Source: CAD feature listing. Evaluate the final solid. Frame: model axes, mm. Face numbers are marked on the shaded views. A direction names the side the tool comes from. Coordinates: 2 decimals unless noted, no trailing zeros. Write each loop counter-clockwise with the first axis right and the second up, starting at its lowest first coordinate (ties: lowest second). Pieces come first, ordered by that corner, then holes. Notation, with made-up numbers: M -9,-3 L 11,-3 A12 ccw 11,12 Z; hole C -35.75,35 d2. An arc over 180 degrees is marked long. One line per item, written item: value. Start each with the question number.
Item 1: Pin query (flat end, axial travel): P1, Ø16, axis at x = -87.5, z = -8.5, coming from the +Y side; P2, Ø4, axis at x = -16.5, y = -41, coming from the +Z side; P3, Ø10, axis at y = -73.5, z = -13, coming from the -X side. Return the tip coordinate at first contact, or that it passes through.
Item 2: Mould query, pull axis X, two halves, no side actions, for the marked faces 5, 6 and 7. Classes: released by +X, released by -X, zero draft, split by the parting line, or undercut.
Item 3: Cut plane C-C, the plane y = -43.5. Output: boundary loops of the cut face in (x, z).
Item 4: Set-up query: the marked faces 1, 2, 3 and 4. Return all of +Z, -Z, +X, -X, +Y, -Y with unobstructed straight access to the full face (end or side cutting, diameter ignored); none if empty.
Item 5: Cut plane A-A, the plane z = 20. Output: boundary loops of the cut face in (x, y).
Item 6: Ray query, L1, parallel to Z at x = -65, y = -5.5; L2, parallel to Z at x = -65, y = -4; L3, parallel to Z at x = -113.5, y = -14. Return the intervals inside material, ascending. Write a range as from..to.
Item 7: Cut plane D-D, the plane x = -113. Output: boundary loops of the cut face in (y, z), then the cut area to 3 significant figures.
Item 8: Cut plane B-B, the plane x = -88. Output: boundary loops of the cut face in (y, z), then the cut area to 3 significant figures.
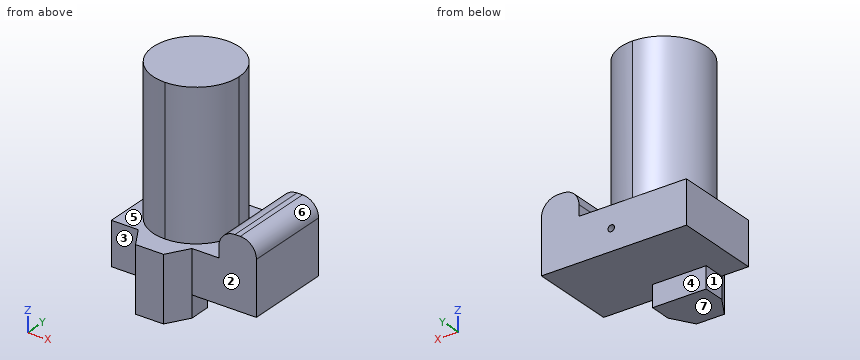
```python
from build123d import *

# Parameters (mm, degrees)
F1_DEPTH = 80
F3_DEPTH = 135
F5_DEPTH = 60
F6_R     = 3
F7_DEPTH = 10


# Not quite as in the source:
# - a feature names something its author has since deleted; it is built from what else it names


with BuildPart() as f1:
    # F0 (on Front) → F1 (new body)
    with BuildSketch(Plane.XZ):
        with BuildLine():
            Line((-135, 0), (0, 0))
            Line((0, 0), (0, 50))
            ThreePointArc((0, 50), (-4.3933982822, 60.6066017178), (-15, 65))
            Line((-15, 65), (-20, 65))
            ThreePointArc((-20, 65), (-30.6066017178, 60.6066017178), (-35, 50))
            Line((-35, 50), (-35, 40))
            Line((-35, 40), (-135, 40))
            Line((-135, 40), (-135, 0))
        make_face()
    extrude(amount=F1_DEPTH)

    # F2 (on face) → F3 (join)
    with BuildSketch(Plane.XY.offset(40)):
        with BuildLine():
            ThreePointArc((-45, -40), (-56.7157287525, -11.7157287525), (-85, 0))
            ThreePointArc((-85, 0), (-125, -40), (-85, -80))
            ThreePointArc((-85, -80), (-56.7157287525, -68.2842712475), (-45, -40))
        make_face()
    extrude(amount=F3_DEPTH)

    # F4 (on face) → F5 (join)
    with BuildSketch(Plane.XY.offset(40)):
        with BuildLine():
            Line((-60, -60), (-110, -60))
            Line((-110, -60), (-110, -71.224989992))
            ThreePointArc((-110, -71.224989992), (-98.247648854, -77.7425462819), (-85, -80))
            ThreePointArc((-85, -80), (-71.7523511459, -77.7425462819), (-60, -71.224989992))
            Line((-60, -71.224989992), (-60, -60))
        make_face()
        with BuildLine():
            ThreePointArc((-85, -80), (-98.247648854, -77.7425462819), (-110, -71.224989992))
            Line((-110, -71.224989992), (-110, -80))
            Line((-110, -80), (-98, -100))
            Line((-98, -100), (-72, -100))
            Line((-72, -100), (-60, -80))
            Line((-60, -80), (-85, -80))
        make_face()
        with BuildLine():
            Line((-60, -80), (-60, -71.224989992))
            ThreePointArc((-60, -71.224989992), (-71.7523511459, -77.7425462819), (-85, -80))
            Line((-85, -80), (-60, -80))
        make_face()
    extrude(amount=-F5_DEPTH)

    # F6 (on face) → F7 (cut)
    with BuildSketch(Plane(origin=(0, 0, 0), x_dir=(-1, 0, 0), z_dir=(0, 1, 0))):
        with Locations((65, 20)):
            Circle(F6_R)
    extrude(amount=-F7_DEPTH, mode=Mode.SUBTRACT)


solid = f1.part
```
From the geometry:
1. P1: stops at y = -60
1. P2: stops at z = 65
1. P3: stops at x = -110
2. face 5: undercut
2. face 6: released by +X
2. face 7: zero draft
3. outline: M -135,0 L 0,0 L 0,50 A15 ccw -15,65 L -20,65 A15 ccw -35,50 L -35,40 L -45.15,40 L -45.15,175 L -124.85,175 L -124.85,40 L -135,40 Z
4. face 1: -Z, -X, +Y, -Y
4. face 2: +Z, -Z, +X, -Y
4. face 3: +Z, -Z, -X, -Y
4. face 4: -Z, +X, -X, +Y
5. outline: M -135,-80 L -110,-80 L -98,-100 L -72,-100 L -60,-80 L 0,-80 L 0,0 L -62,0 L -62,-10 L -68,-10 L -68,0 L -135,0 Z
6. L1: z = 0..17, 23..175
6. L2: z = 0..17, 23..40
6. L3: z = 0..175
7. outline: M -80,0 L 0,0 L 0,40 L -11.43,40 L -11.43,175 L -68.57,175 L -68.57,40 L -80,40 Z
7. area: 10,900 mm²
8. outline: M -100,-20 L -60,-20 L -60,0 L 0,0 L 0,40 L -0.11,40 L -0.11,175 L -79.89,175 L -79.89,40 L -100,40 Z
8. area: 15,600 mm²
